Build history of the part. All positions in model axes, mm. Face numbers are marked on the shaded views. A direction names the side the tool comes from. Give positions to 0.01 mm unless a question says otherwise; leave off trailing zeros. Order: outer loops, then holes, each group sorted by start corner. A loop starts at its lowest first (then second) coordinate and runs counter-clockwise, first axis right, second up. Notation, with made-up numbers: (22.25, -17.75) - (45.25, -17.75) arc R26 ccw to (45.25, -0.75) - close; hole circle Ø3 at (54, 28). An arc over 180 degrees is marked (long way). Use a Markdown table: item, result. Add a question column.
(1) Slice it at C-C (z = 9.75). Write the cut outline in (x, y).
(2) Slice it at D-D (x = 23). Write the cut outline in (y, z).
(3) Slice it at B-B (x = 15). Write the cut outline in (y, z).
(4) Which spindle directions (+Z, -Z, +X, -X, +Y, -Y) get a long thin tool onto all of the face, cutting with end or side? Do the marked faces 4, 5 and 6. Say none if no direction does.
(5) Mould opens along Y. For the marked faces 1, 2 and 3 say: +Y half, -Y half, draft (parallel to the pull), parting line (faces both ways), or undercut.
(6) Flat gauge pins, fed straight in: pin 1 (8 mm diameter, centred on y = -12, z = 15.5, fed in from +X); pin 2 (1 mm diameter, centred on y = -5.5, z = 21.5, fed in from +X); pin 3 (5 mm diameter, centred on x = 40, z = 8, fed in from -Y); pin 4 (2.5 mm diameter, centred on x = 12.5, y = -1.5, fed in from +Z). Where does each tip first touch, or does it go through?
(7) Wall check: line 1 (X direction, y = -12.6, z = 8); line 2 (Y direction, x = 29.5, z = 19.25); line 3 (Y direction, x = 30, z = 21.15). Give the ranges that are in metal, low to high.
(8) Slice it at A-A (y = -7). Write the cut outline in (x, z).
from build123d import *

# Parameters (mm, degrees)
F0_R           = 3
F0_W           = 20
F0_H           = 8
F1_DEPTH       = 14
F2_R           = 7.99999
F3_W           = 62.9811411479
F3_H           = 8
F4_DEPTH       = 21
F6_D           = 5.5
F6_CSINK_D     = 11.2
F6_CSINK_ANGLE = 90


# Not quite as in the source:
# - a fillet or chamfer is up to 0.001 mm smaller than in the source, because OpenCascade refuses the exact size


with BuildPart() as f1:
    # F0 (on Front) → F1 (new body)
    with BuildSketch(Plane.XZ):
        Polygon((0, 16), (0, 0), (48, 0), (48, 16), (40, 16), (20, 16), align=None)
        with Locations((8, 8)):
            Circle(F0_R, mode=Mode.SUBTRACT)
        with Locations((40, 8)):
            Circle(F0_R, mode=Mode.SUBTRACT)
        with Locations((30, 20)):
            Rectangle(F0_W, F0_H)
    extrude(amount=F1_DEPTH)

    # F2 (radius 8 in the source; OpenCascade refuses exactly that, so slightly less here)
    f2_edges = [f1.edges().sort_by_distance(p)[0] for p in [
        (0, -7, 16),
        (0, -7, 0),
        (48, -7, 16),
        (48, -7, 0),
    ]]
    fillet(f2_edges, radius=F2_R)

    # F3 (on face) → F4 (cut)
    with BuildSketch(Plane(origin=(0, 0, 0), x_dir=(1, 0, 0), z_dir=(0, 0, -1))):
        with Locations((30.1177082001, 7)):
            Rectangle(F3_W, F3_H)
    extrude(amount=-F4_DEPTH, mode=Mode.SUBTRACT)

    # F6 (through all)
    with Locations(Plane.XY.offset(24)):
        with Locations((30, -7)):
            CounterSinkHole(F6_D / 2, F6_CSINK_D / 2, counter_sink_angle=F6_CSINK_ANGLE)


solid = f1.part
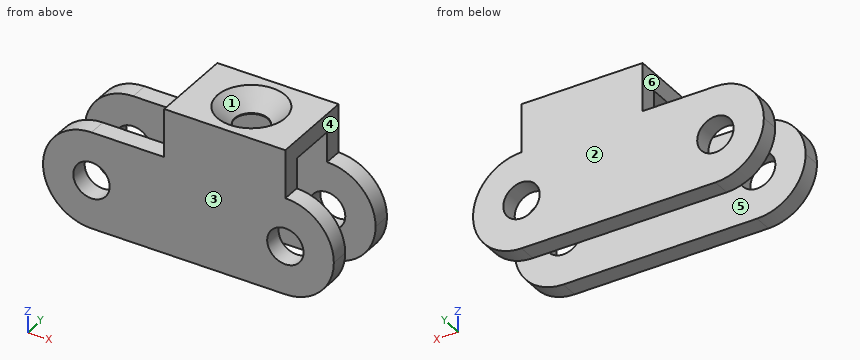
Solution:
| question | item | result |
|---|---|---|
| 1 | outline | (0.19, -14) - (5.56, -14) - (5.56, -11) - (0.19, -11) - close; (0.19, -3) - (5.56, -3) - (5.56, 0) - (0.19, 0) - close; (10.44, -14) - (37.56, -14) - (37.56, -11) - (10.44, -11) - close; (10.44, -3) - (37.56, -3) - (37.56, 0) - (10.44, 0) - close; (42.44, -14) - (47.81, -14) - (47.81, -11) - (42.44, -11) - close; (42.44, -3) - (47.81, -3) - (47.81, 0) - (42.44, 0) - close |
| 2 | outline | (-14, 0) - (-11, 0) - (-11, 21) - (-3, 21) - (-3, 0) - (0, 0) - (0, 24) - (-14, 24) - close |
| 3 | outline | (-14, 0) - (-11, 0) - (-11, 16) - (-14, 16) - close; (-3, 0) - (0, 0) - (0, 16) - (-3, 16) - close |
| 4 | face 4 | +Z, +X, +Y, -Y |
| 4 | face 5 | -Z, +X, -X |
| 4 | face 6 | +Z, -X, +Y, -Y |
| 5 | face 1 | undercut |
| 5 | face 2 | +Y half |
| 5 | face 3 | -Y half |
| 6 | pin 1 | x = 47.19 |
| 6 | pin 2 | x = 40 |
| 6 | pin 3 | through |
| 6 | pin 4 | z = 16 |
| 7 | line 1 | 0 to 5, 11 to 37, 43 to 48 |
| 7 | line 2 | -14 to -11, -3 to 0 |
| 7 | line 3 | -14 to -9.75, -4.25 to 0 |
| 8 | outline | (20, 21) - (27.25, 21) - (27.25, 21.15) - (24.4, 24) - (20, 24) - close; (32.75, 21) - (40, 21) - (40, 24) - (35.6, 24) - (32.75, 21.15) - close |
